Part model, mm, in its own coordinate system. A direction names the side the tool comes from. Coordinates: 2 decimals unless noted, no trailing zeros. Order: outer loops, then holes, each group sorted by start corner. A loop starts at its lowest first (then second) coordinate and runs counter-clockwise, first axis right, second up.
from build123d import *
from OCP.BRepFilletAPI import BRepFilletAPI_MakeChamfer

# Parameters (mm, degrees)
SKETCH1_W               = 29.5
SKETCH1_H               = 29.5
BOSS_EXTRUDE1_DEPTH     = 16
SKETCH2_R               = 12.75
CUT_EXTRUDE1_DEPTH      = 13.5
CHAMFER1_SIZE           = 22.860104606
CHAMFER1_SIZE_2         = 2
CHAMFER2_SIZE           = 4
CHAMFER2_SIZE2          = 4.030734246
SKETCH5_R               = 10
CUT_EXTRUDE2_DEPTH      = 10
BOSS_EXTRUDE2_START     = -1
BOSS_EXTRUDE2_DEPTH     = 1
MIRROR2_START           = -1
MIRROR2_COPY_1_DEPTH    = 1
CUT_EXTRUDE3_DEPTH      = 45.646312331
CUT_EXTRUDE3_DEPTH_BACK = 45.646312331
SKETCH7_R               = 1.125
SKETCH8_R               = 1
CUT_EXTRUDE4_DEPTH      = 45.992146034
SKETCH17_R              = 1.5
CUT_EXTRUDE12_DEPTH     = 13.5
SKETCH11_OUTSIDE_W      = 41.044
SKETCH11_OUTSIDE_H      = 41.014
SKETCH11_OUTSIDE_R      = 19
CUT_EXTRUDE6_DEPTH      = 45.992146034
SKETCH12_R              = 2
CUT_EXTRUDE7_DEPTH      = 15
SKETCH13_W              = 11
SKETCH13_H              = 30.855989766
CUT_EXTRUDE8_DEPTH      = 7
CUT_EXTRUDE9_DEPTH      = 45.557331201
CUT_EXTRUDE9_DEPTH_BACK = 45.557331201
SKETCH14_W              = 11
SKETCH14_H              = 9.5
BOSS_EXTRUDE4_START     = -4
BOSS_EXTRUDE4_DEPTH     = 4


with BuildPart() as part:
    # Sketch1 → Boss-Extrude1 (new body)
    with BuildSketch(Plane(origin=(0, 0, 0), x_dir=(1, 0, 0), z_dir=(0, 1, 0))):
        with Locations((14.75, 14.75)):
            Rectangle(SKETCH1_W, SKETCH1_H)
    extrude(amount=BOSS_EXTRUDE1_DEPTH)

    # Sketch2 → Cut-Extrude1 (cut)
    with BuildSketch(Plane(origin=(0, 16, 0), x_dir=(1, 0, 0), z_dir=(0, 1, 0))):
        with Locations(Location((14.75, 14.75, 0), (0, 0, 270))):
            Circle(SKETCH2_R)
    extrude(amount=-CUT_EXTRUDE1_DEPTH, mode=Mode.SUBTRACT)

    # Chamfer1
    # the kernel refuses this chamfer: 22.860104606, 2 mm, written as the material it takes off along each edge
    with BuildSketch(Plane(origin=(-59.427907001, 0, 0), x_dir=(0, 1, 0), z_dir=(1, 0, 0)), Plane(origin=(29.5, 0, 59.427907001), x_dir=(0, 1, 0), z_dir=(0, 0, -1)), Plane(origin=(0, 0, -88.927907001), x_dir=(0, 1, 0), z_dir=(0, 0, 1))) as chamfer1_piece_1:
        Polygon((CHAMFER1_SIZE, 0), (0, -CHAMFER1_SIZE_2), (0, 0), align=None)
    extrude(amount=148.355814002, mode=Mode.SUBTRACT)
    with BuildSketch(Plane(origin=(88.927907001, 0, -29.5), x_dir=(0, 0, 1), z_dir=(-1, 0, 0))) as chamfer1_piece_2:
        Polygon((CHAMFER1_SIZE_2, 0), (0, CHAMFER1_SIZE), (0, 0), align=None)
    extrude(amount=148.355814002, mode=Mode.SUBTRACT)

    # Chamfer2: one chamfer whose edges measure the first distance from different faces: ONE call of the kernel's chamfer builder (chamfer() names one face for all edges)
    chamfer2_edges_1 = [part.edges().sort_by_distance(p)[0] for p in [
        (1.300090692, 8, -28.199909308),
        (28.199909308, 8, -28.199909308),
    ]]
    chamfer2_side_1 = [part.faces().sort_by_distance(p)[0] for p in [
        (14.75, 8.13876858, -28.212049986),
    ]]
    chamfer2_edges_2 = [part.edges().sort_by_distance(p)[0] for p in [
        (1.300090692, 8, -1.300090692),
    ]]
    chamfer2_side_2 = [part.faces().sort_by_distance(p)[0] for p in [
        (1.287950014, 8.13876858, -14.75),
    ]]
    chamfer2_edges_3 = [part.edges().sort_by_distance(p)[0] for p in [
        (28.199909308, 8, -1.300090692),
    ]]
    chamfer2_side_3 = [part.faces().sort_by_distance(p)[0] for p in [
        (28.212049986, 8.13876858, -14.75),
    ]]
    chamfer2 = BRepFilletAPI_MakeChamfer(part.part.solid().wrapped)
    for e in chamfer2_edges_1:
        chamfer2.Add(CHAMFER2_SIZE, CHAMFER2_SIZE2, e.wrapped, chamfer2_side_1[0].wrapped)  # the first distance lies on this face
    for e in chamfer2_edges_2:
        chamfer2.Add(CHAMFER2_SIZE, CHAMFER2_SIZE2, e.wrapped, chamfer2_side_2[0].wrapped)  # the first distance lies on this face
    for e in chamfer2_edges_3:
        chamfer2.Add(CHAMFER2_SIZE, CHAMFER2_SIZE2, e.wrapped, chamfer2_side_3[0].wrapped)  # the first distance lies on this face
    add(Compound.cast(chamfer2.Shape()), mode=Mode.REPLACE)

    # Sketch5 → Cut-Extrude2 (cut)
    with BuildSketch(Plane.XZ):
        with Locations(Location((14.75, -14.734574622, 0), (0, 0, 270))):
            Circle(SKETCH5_R)
    extrude(amount=-CUT_EXTRUDE2_DEPTH, mode=Mode.SUBTRACT)

    # Boss-Extrude2: read off the stored shape, not the designer's step
    # Boss-Extrude2 outline → Boss-Extrude2 (add)
    with BuildSketch(Plane(origin=(0, 16, 0), x_dir=(1, 0, 0), z_dir=(0, 1, 0)).offset(BOSS_EXTRUDE2_START)):
        with BuildLine():
            Line((0.600181384, 4.615344889), (4.646195644, 0.600181384))
            Line((4.646195644, 0.600181384), (24.853804356, 0.600181384))
            Line((24.853804356, 0.600181384), (28.899818616, 4.615344889))
            Line((28.899818616, 4.615344889), (28.899818616, 24.853804356))
            Line((28.899818616, 24.853804356), (24.884655111, 28.899818616))
            Line((24.884655111, 28.899818616), (4.615344889, 28.899818616))
            ThreePointArc((4.615344889, 28.899818616), (0.584756006, 28.884393239), (0.600181384, 24.853804356))
            Line((0.600181384, 24.853804356), (0.600181384, 4.615344889))
        make_face()
        Polygon((24.797166447, 28.812329953), (28.812329953, 24.766315692), (28.812329953, 4.702833553), (24.766315692, 0.687670047), (4.733684308, 0.687670047), (0.687670047, 4.702833553), (0.687670047, 24.766315692), (4.702833553, 28.812329953), align=None, mode=Mode.SUBTRACT)
    boss_extrude2 = extrude(amount=BOSS_EXTRUDE2_DEPTH)

    # Mirror1: Boss-Extrude2 across plane
    add(boss_extrude2.mirror(Plane(origin=(14.75, 0, 0), x_dir=(0, 0, 1), z_dir=(1, 0, 0))))

    # Mirror2: Boss-Extrude2 across plane
    add(boss_extrude2.mirror(Plane.XY.offset(-14.75)))

    # Mirror2 copy 1 sketch → Mirror2 copy 1 (add)
    with BuildSketch(Plane(origin=(29.5, 16, -29.5), x_dir=(-1, 0, 0), z_dir=(0, 1, 0)).offset(MIRROR2_START)):
        with BuildLine():
            Line((0.600181384, 4.615344889), (4.646195644, 0.600181384))
            Line((4.646195644, 0.600181384), (24.853804356, 0.600181384))
            Line((24.853804356, 0.600181384), (28.899818616, 4.615344889))
            Line((28.899818616, 4.615344889), (28.899818616, 24.853804356))
            Line((28.899818616, 24.853804356), (24.884655111, 28.899818616))
            Line((24.884655111, 28.899818616), (4.615344889, 28.899818616))
            ThreePointArc((4.615344889, 28.899818616), (0.584756006, 28.884393239), (0.600181384, 24.853804356))
            Line((0.600181384, 24.853804356), (0.600181384, 4.615344889))
        make_face()
        Polygon((24.797166447, 28.812329953), (28.812329953, 24.766315692), (28.812329953, 4.702833553), (24.766315692, 0.687670047), (4.733684308, 0.687670047), (0.687670047, 4.702833553), (0.687670047, 24.766315692), (4.702833553, 28.812329953), align=None, mode=Mode.SUBTRACT)
    extrude(amount=MIRROR2_COPY_1_DEPTH)

    # Sketch7 → Cut-Extrude3 (cut, two sides: drawn at the far end of the back side and taken through both)
    with BuildSketch(Plane.XZ.offset(-15).offset(-CUT_EXTRUDE3_DEPTH_BACK)):
        with Locations(Location((2.607763136, -2.623188514, 0), (0, 0, 270))):
            Circle(SKETCH7_R)
        with Locations(Location((26.892236864, -2.623188514, 0), (0, 0, 308.909428046))):
            Circle(SKETCH7_R)
        with Locations(Location((26.892236864, -26.876811486, 0), (0, 0, 270))):
            Circle(SKETCH7_R)
        with Locations(Location((2.607763136, -26.876811486, 0), (0, 0, 270))):
            Circle(SKETCH7_R)
    extrude(amount=CUT_EXTRUDE3_DEPTH + CUT_EXTRUDE3_DEPTH_BACK, mode=Mode.SUBTRACT)

    # Sketch8 → Cut-Extrude4 (cut, through all)
    with BuildSketch(Plane.XZ):
        with Locations(Location((7.58, -4.521537889, 0), (0, 0, 270))):
            Circle(SKETCH8_R)
        with Locations(Location((4.219388969, -9.118549755, 0), (0, 0, 270))):
            Circle(SKETCH8_R)
        with Locations(Location((7.604770426, -24.995781156, 0), (0, 0, 270))):
            Circle(SKETCH8_R)
        with Locations(Location((21.944728448, -24.96108318, 0), (0, 0, 270))):
            Circle(SKETCH8_R)
        with Locations(Location((25.294206418, -20.355953224, 0), (0, 0, 270))):
            Circle(SKETCH8_R)
        with Locations(Location((21.92, -4.521537889, 0), (0, 0, 270))):
            Circle(SKETCH8_R)
        with Locations(Location((3.375033299, -14.777523673, 0), (0, 0, 90))):
            Circle(SKETCH8_R)
        with Locations(Location((4.233046011, -20.406914295, 0), (0, 0, 245.746224718))):
            Circle(SKETCH8_R)
        with Locations(Location((26.125, -14.75, 0), (0, 0, 90))):
            Circle(SKETCH8_R)
        with Locations(Location((25.280611031, -9.118549755, 0), (0, 0, 350.665442319))):
            Circle(SKETCH8_R)
    extrude(amount=-CUT_EXTRUDE4_DEPTH, mode=Mode.SUBTRACT)

    # Sketch17 → Cut-Extrude12 (cut)
    with BuildSketch(Plane(origin=(0, 2.5, 0), x_dir=(1, 0, 0), z_dir=(0, 1, 0))):
        with Locations((7.604770426, 24.995781156)):
            Circle(SKETCH17_R)
        with Locations((4.233046011, 20.406914295)):
            Circle(SKETCH17_R)
        with Locations((4.219388969, 9.118549755)):
            Circle(SKETCH17_R)
        with Locations((7.58, 4.521537889)):
            Circle(SKETCH17_R)
        with Locations((21.92, 4.521537889)):
            Circle(SKETCH17_R)
        with Locations((25.280611031, 9.118549755)):
            Circle(SKETCH17_R)
        with Locations((25.294206418, 20.355953224)):
            Circle(SKETCH17_R)
        with Locations((21.944728448, 24.96108318)):
            Circle(SKETCH17_R)
    extrude(amount=CUT_EXTRUDE12_DEPTH, mode=Mode.SUBTRACT)

    # Sketch11 outside → Cut-Extrude6 (cut, through all)
    with BuildSketch(Plane.XZ):
        with Locations((14.75, -14.75)):
            Rectangle(SKETCH11_OUTSIDE_W, SKETCH11_OUTSIDE_H)
        with Locations((14.75, -14.734574622)):
            Circle(SKETCH11_OUTSIDE_R, mode=Mode.SUBTRACT)
    extrude(amount=-CUT_EXTRUDE6_DEPTH, mode=Mode.SUBTRACT)

    # Sketch12 → Cut-Extrude7 (cut)
    with BuildSketch(Plane.XZ):
        with Locations((2.607763136, -2.623188514)):
            Circle(SKETCH12_R)
        with Locations((26.892236864, -2.623188514)):
            Circle(SKETCH12_R)
        with Locations((26.892236864, -26.876811486)):
            Circle(SKETCH12_R)
        with Locations((2.607763136, -26.876811486)):
            Circle(SKETCH12_R)
    extrude(amount=-CUT_EXTRUDE7_DEPTH, mode=Mode.SUBTRACT)

    # Sketch13 → Cut-Extrude8 (cut)
    with BuildSketch(Plane.XZ):
        with Locations((14.75, -15.427994883)):
            Rectangle(SKETCH13_W, SKETCH13_H)
    extrude(amount=-CUT_EXTRUDE8_DEPTH, mode=Mode.SUBTRACT)

    # Sketch14 → Cut-Extrude9 (cut, two sides: drawn at the far end of the back side and taken through both)
    with BuildSketch(Plane(origin=(0.600181384, 0, 0), x_dir=(0, 0, -1), z_dir=(1, 0, 0)).offset(-CUT_EXTRUDE9_DEPTH_BACK)):
        with Locations((14.747577474, 7.25)):
            Rectangle(SKETCH14_W, SKETCH14_H)
    extrude(amount=CUT_EXTRUDE9_DEPTH + CUT_EXTRUDE9_DEPTH_BACK, mode=Mode.SUBTRACT)

    # Boss-Extrude4: read off the stored shape, not the designer's step
    # Boss-Extrude4 outline → Boss-Extrude4 (add)
    with BuildSketch(Plane(origin=(0, 11, 0), x_dir=(1, 0, 0), z_dir=(0, 1, 0)).offset(BOSS_EXTRUDE4_START)):
        with BuildLine():
            Line((26.775051343, 9.247577474), (24.274880385, 9.247577474))
            ThreePointArc((24.274880385, 9.247577474), (14.75, 3.75), (5.225119615, 9.247577474))
            Line((5.225119615, 9.247577474), (2.724948657, 9.247577474))
            ThreePointArc((2.724948657, 9.247577474), (3.101034316, 8.118908385), (4.18060697, 7.619051187))
            ThreePointArc((4.18060697, 7.619051187), (5.146820144, 6.363019814), (6.261378349, 5.236546239))
            ThreePointArc((6.261378349, 5.236546239), (6.718994568, 3.293258749), (8.701845126, 3.52581528))
            ThreePointArc((8.701845126, 3.52581528), (14.75, 2), (20.798154874, 3.52581528))
            ThreePointArc((20.798154874, 3.52581528), (22.781005432, 3.293258749), (23.238621651, 5.236546239))
            ThreePointArc((23.238621651, 5.236546239), (24.353179856, 6.363019814), (25.31939303, 7.619051187))
            ThreePointArc((25.31939303, 7.619051187), (26.398965684, 8.118908385), (26.775051343, 9.247577474))
        make_face()
        with BuildLine():
            Line((24.277677677, 20.247577474), (26.790286194, 20.247577474))
            ThreePointArc((26.790286194, 20.247577474), (26.406849135, 21.361948346), (25.336616586, 21.855353563))
            ThreePointArc((25.336616586, 21.855353563), (24.373445414, 23.11371917), (23.261616159, 24.242886303))
            ThreePointArc((23.261616159, 24.242886303), (22.808703381, 26.187275382), (20.825295919, 25.959517362))
            ThreePointArc((20.825295919, 25.959517362), (14.78085071, 27.499962676), (8.729021582, 25.988786362))
            ThreePointArc((8.729021582, 25.988786362), (6.746739537, 26.226140044), (6.284422555, 24.28396552))
            ThreePointArc((6.284422555, 24.28396552), (5.167141926, 23.160192099), (4.197892408, 21.906502313))
            ThreePointArc((4.197892408, 21.906502313), (3.105798999, 21.396517333), (2.74153276, 20.247577474))
            Line((2.74153276, 20.247577474), (5.222322323, 20.247577474))
            ThreePointArc((5.222322323, 20.247577474), (14.75, 25.75), (24.277677677, 20.247577474))
        make_face()
    extrude(amount=BOSS_EXTRUDE4_DEPTH)


solid = part.part
Q1. Which spindle directions (+Z, -Z, +X, -X, +Y, -Y) get a long thin tool onto all of the face, cutting with end or side? Do faces 1 (the face through (16, 11, -26)), 2 (the face through (22.76, 4.72, -3.28)), 3 (the face through (25.5, 9.06, -25.44)). Say none if no direction does.
Results list:
face 1: +Y
face 2: none
face 3: -Y
Q2. Cut at A-A on y = 9.5. Write the cut outline in (x, z).
Results list:
outline: (1.17, -24.29) - (1.89, -25.01) arc R2 cw to (4.47, -27.61) - (5.18, -28.33) - (24.32, -28.33) - (25.03, -27.61) arc R2 cw to (27.61, -25.01) - (28.33, -24.29) - (28.33, -20.25) - (24.28, -20.25) arc R11 cw to (5.22, -20.25) - (1.17, -20.25) - close; (1.17, -9.25) - (5.23, -9.25) arc R11 cw to (24.27, -9.25) - (28.33, -9.25) - (28.33, -5.18) - (27.63, -4.48) arc R2 cw to (25.03, -1.9) - (24.29, -1.17) - (5.21, -1.17) - (4.47, -1.9) arc R2 cw to (1.87, -4.48) - (1.17, -5.18) - close
Q3. Pin check, flat tips, straight feed: pin 1 Ø2.5 at (x, z) = (21.94, -24.96) entering from +Y; pin 2 Ø2 at (y, z) = (12.5, -15) entering from +X; pin 3 Ø1.8 at (x, z) = (26.89, -2.62) entering from +Y; pin 4 Ø5 at (y, z) = (2, -5) entering from +X. Stop position of each tip, or through.
Results list:
pin 1: stops at y = 11
pin 2: stops at x = 28.68
pin 3: passes through
pin 4: stops at x = 27.89
Q4. Cut at C-C on x = 12.5. Write the cut outline in (y, z), and give its area (3 significant figures).
Results list:
outline: (7, -28.11) - (15, -28.81) - (15, -28.9) - (16, -28.9) - (16, -27.3) - (11, -27.3) - (11, -25.52) - (7, -25.52) - close; (7, -3.98) - (11, -3.98) - (11, -2.2) - (16, -2.2) - (16, -0.6) - (15, -0.6) - (15, -0.69) - (7, -1.39) - close
area: 36.1 mm2
Q5. Mould opens along X. For faces 4 (the face through (3.331, 1.232, -15.777)), 5 (the face through (14.5, 16, -1.7)), 6 (the face through (27.529, 5.938, -24.468)) say: pulls with the +X half, pulls with the -X half, needs draft (parallel to the pull), parting line crosses it, or undercut.
Results list:
face 4: undercut
face 5: needs draft
face 6: pulls with the +X half
Q6. Cut at B-B on z = -14.75. Write the cut outline in (x, y) (3 decimals).
Results list:
outline: (0.6, 15) - (0.688, 15) - (0.95, 12) - (2, 12) - (2, 16) - (0.6, 16) - close; (1.781, 2.5) - (2, 0) - (2.375, 0) - (2.375, 2.5) - close; (4.375, 0) - (4.75, 0) - (4.75, 2.5) - (4.375, 2.5) - close; (24.75, 0) - (25.125, 0) - (25.125, 2.5) - (24.75, 2.5) - close; (27.125, 0) - (27.5, 0) - (27.719, 2.5) - (27.125, 2.5) - close; (27.5, 12) - (28.55, 12) - (28.812, 15) - (28.9, 15) - (28.9, 16) - (27.5, 16) - close
Q7. Wall check: line 1 along Z through (x, y) = (21.5, 1.25); line 2 along Y through (x, z) = (26.75, -16.75); line 3 along Z through (x, y) = (3.5, 15.25). Give the ranges that are in metal, low to high.
Results list:
line 1: z = -27.61 to -25.86, -24.07 to -22.11, -7.36 to -5.43, -3.61 to -1.89
line 2: y = 0 to 2.5
line 3: z = -29.58 to -27.56, -26.19 to -21.72, -7.8 to -3.31, -1.94 to 0.08
